Autodesk Inventor part; units mm, degrees
ref_plane "YZ Plane" through (0, 0, 0) normal (1, 0, 0) x (0, 1, 0)
ref_plane "XZ Plane" through (0, 0, 0) normal (0, 1, 0) x (-1, 0, 0)
ref_plane "XY Plane" through (0, 0, 0) normal (0, 0, 1) x (1, 0, 0)
sketch "Sketch1" plane through (0, 0, 0) normal (0, 0, 1) x (1, 0, 0)
  line L0 (0, 0) -> (0, 15.875)
  line L1 (0, 15.875) -> (0.7937, 15.875)
  line L2 (0.7937, 15.875) -> (0.7938, 0.7937)
  line L3 (0.7938, 0.7937) -> (15.875, 0.7937)
  line L4 (15.875, 0.7937) -> (15.875, 0)
  line L5 (15.875, 0) -> (0, 0)
  dimension "d0" = 15.875
  dimension "d1" = 0.7937
extrude "Extrusion1" add sketch "Sketch1" along normal blind 292.1
sketch "Sketch2" plane through (0.7938, 0.7937, 0) normal (0, 1, 0) x (1, 0, 0)
  line L0 (0, 0) -> (15.0812, 0)
  line L1 (15.0812, -292.1) -> (0, -292.1)
  line L2 (7.5406, 0) -> (7.5406, -292.1) construction
  circle A0 centre (7.5406, -6.35) radius 1.5875
  circle A1 centre (7.5406, -76.2) radius 1.5875
  circle A2 centre (7.5406, -146.05) radius 1.5875
  circle A3 centre (7.5406, -215.9) radius 1.5875
  circle A4 centre (7.5406, -285.75) radius 1.5875
  point P0 (-0.7938, 0)
  dimension "d4" = 6.35
  dimension "d5" = 3.175
  dimension "d6" = 292.1
  dimension "d9" = 69.85
sketch "Sketch3" plane through (0.7938, 0.7937, 0) normal (1, 0, 0) x (0, 0, -1)
  line L0 (0, 15.0812) -> (0, 0)
  line L1 (-292.1, 0) -> (-292.1, 15.0812)
  line L2 (-292.1, 7.5406) -> (0, 7.5406) construction
  circle A0 centre (-12.7, 7.5406) radius 1.5875
  circle A1 centre (-79.375, 7.5406) radius 1.5875
  circle A2 centre (-146.05, 7.5406) radius 1.5875
  circle A3 centre (-212.725, 7.5406) radius 1.5875
  circle A4 centre (-279.4, 7.5406) radius 1.5875
  point P0 (0, -0.7937)
  dimension "d14" = 3.175
  dimension "d15" = 12.7
  dimension "d16" = 292.1
  dimension "d19" = 66.675
extrude "Extrusion2" cut sketch "Sketch2" against normal through all
extrude "Extrusion3" cut sketch "Sketch3" against normal through all
equation "\"d9\" = -0.5 * d4 + 0.25 * d6"
equation "\"d19\" = -0.5 * d15 + 0.25 * d16"
properties part number "Hopper Bracing Top Left P4" material "Aluminum 6061"
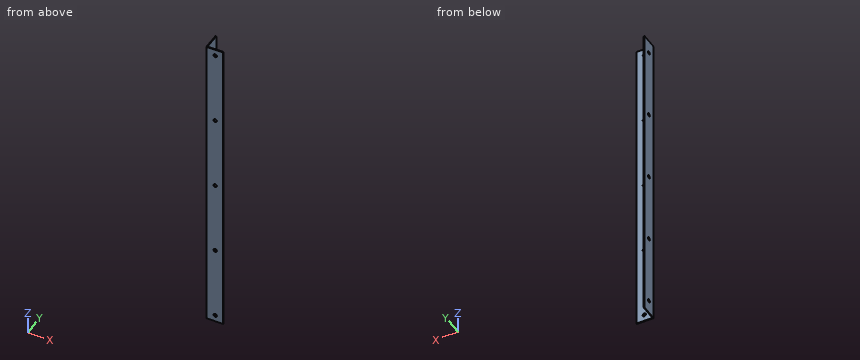
Geometry: final body of the model. Coordinates: model frame, mm. Give positions to 0.01 mm unless a question says otherwise; leave off trailing zeros. Loops run counter-clockwise (first coordinate to the right, second up) from the corner with the lowest first, then second, coordinate; pieces in that order, holes last. Notation, with made-up numbers: (-29.5, 73) -> (17.5, 73) arc R26 ccw to (17.5, 102) -> close; hole circle Ø5 at (66, 30.25). An arc over 180 degrees is marked (long way). Return JSON: item names as keys, results as strings.
Item 1: Pin query (flat end, axial travel): P1, Ø2, axis at x = 9.5, z = 257, coming from the +Y side; P2, Ø8, axis at y = 8, z = 83, coming from the +X side. Return the tip coordinate at first contact, or that it passes through.
Filled in:
{"P1": "y = 0.79", "P2": "x = 0.79"}
Item 2: Line query: line 1 (X direction, y = 0.5, z = 76.2) (3 decimals); line 2 (Y direction, x = 3.5, z = 197). Output: solid intervals per line, ascending.
Filled in:
{"line 1": "0 to 6.747, 9.922 to 15.875", "line 2": "0 to 0.79"}
Item 3: Section A-A, the plane z = 45.5. Output: boundary loops of the cut face in (x, y) (3 decimals).
Filled in:
{"outline": "(0, 0) -> (15.875, 0) -> (15.875, 0.794) -> (0.794, 0.794) -> (0.794, 15.875) -> (0, 15.875) -> close"}
Item 4: Section B-B, the plane y = 13. Output: boundary loops of the cut face in (x, z).
Filled in:
{"outline": "(0, 0) -> (0.79, 0) -> (0.79, 292.1) -> (0, 292.1) -> close"}
